from build123d import *

# Parameters (mm, degrees)
BOSS_EXTRU_1_DEPTH                              = 8
SKETCH1_R                                       = 3.375
CUT_EXTRUDE1_DEPTH                              = 9
ESQUISSE7_W                                     = 7
ESQUISSE7_H                                     = 3.5
ENL_V_MAT_EXTRU_2_DEPTH                         = 9
CHAMBRAGE_POUR_VIS_T_TE_CYLINDRIQUE_D           = 2.5
CHAMBRAGE_POUR_VIS_T_TE_CYLINDRIQUE_CBORE_D     = 4.5
CHAMBRAGE_POUR_VIS_T_TE_CYLINDRIQUE_CBORE_DEPTH = 5.3
CBORE_FOR_M5_HEX_HEAD_BOLT1_D                   = 4
CBORE_FOR_M5_HEX_HEAD_BOLT1_DEPTH               = 9.499
CBORE_FOR_M5_HEX_HEAD_BOLT1_CBORE_D             = 6.2
CBORE_FOR_M5_HEX_HEAD_BOLT1_CBORE_DEPTH         = 2
CBORE_FOR_M5_HEX_HEAD_BOLT1_TIP                 = 1.201721238


with BuildPart() as part:
    # Esquisse1 → Boss.-Extru.1 (new body)
    with BuildSketch(Plane(origin=(0, 0, 0), x_dir=(1, 0, 0), z_dir=(0, 1, 0))):
        with BuildLine():
            Line((6.025985397, 9.5), (-6.025985397, 9.5))
            ThreePointArc((-6.025985397, 9.5), (0, -11.25), (6.025985397, 9.5))
        make_face()
    extrude(amount=BOSS_EXTRU_1_DEPTH)

    # Sketch1 → Cut-Extrude1 (cut, through all)
    with BuildSketch(Plane(origin=(0, 8, 0), x_dir=(1, 0, 0), z_dir=(0, 1, 0))):
        Circle(SKETCH1_R)
    extrude(amount=-CUT_EXTRUDE1_DEPTH, mode=Mode.SUBTRACT)

    # Esquisse7 → Enlèv. mat.-Extru.2 (cut, through all)
    with BuildSketch(Plane(origin=(0, 8, 0), x_dir=(1, 0, 0), z_dir=(0, 1, 0))):
        with Locations((0, 5.75)):
            Rectangle(ESQUISSE7_W, ESQUISSE7_H)
    extrude(amount=-ENL_V_MAT_EXTRU_2_DEPTH, mode=Mode.SUBTRACT)

    # Chambrage pour vis à tête cylindrique à 6 pans creux (ou vis CHC) M21 (through all)
    with Locations(Plane(origin=(0, 8, 0), x_dir=(1, 0, 0), z_dir=(0, 1, 0))):
        with Locations((-8, 0), (0, -8), (8, 0)):
            CounterBoreHole(CHAMBRAGE_POUR_VIS_T_TE_CYLINDRIQUE_D / 2, CHAMBRAGE_POUR_VIS_T_TE_CYLINDRIQUE_CBORE_D / 2, CHAMBRAGE_POUR_VIS_T_TE_CYLINDRIQUE_CBORE_DEPTH)

    # CBORE for M5 Hex Head Bolt1
    with Locations(Plane(origin=(0, 0, -9.5), x_dir=(-1, 0, 0), z_dir=(0, 0, -1))):
        with Locations((0, 4)):
            CounterBoreHole(CBORE_FOR_M5_HEX_HEAD_BOLT1_D / 2, CBORE_FOR_M5_HEX_HEAD_BOLT1_CBORE_D / 2, CBORE_FOR_M5_HEX_HEAD_BOLT1_CBORE_DEPTH, depth=CBORE_FOR_M5_HEX_HEAD_BOLT1_DEPTH)
            with Locations((0, 0, -(CBORE_FOR_M5_HEX_HEAD_BOLT1_DEPTH + CBORE_FOR_M5_HEX_HEAD_BOLT1_TIP / 2))):  # 118° drill point
                Cone(0, CBORE_FOR_M5_HEX_HEAD_BOLT1_D / 2, CBORE_FOR_M5_HEX_HEAD_BOLT1_TIP, mode=Mode.SUBTRACT)


solid = part.part
Build history of the part. All positions in model axes, mm. A direction names the side the tool comes from. Coordinates: 2 decimals unless noted, no trailing zeros. Order: outer loops, then holes, each group sorted by start corner. A loop starts at its lowest first (then second) coordinate and runs counter-clockwise, first axis right, second up. Notation, with made-up numbers: (2, 17.5) - (38, 17.5) arc R25 ccw to (38, 46.5) - close; hole circle Ø7 at (13.5, 22). An arc over 180 degrees is marked (long way). Write each question's results on one line, items separated by ' | '. Start each with the question number.
Item 1: Flat gauge pins, fed straight in: pin 1 (3.5 mm diameter, centred on x = -7.5, z = 0.5, fed in from +Y); pin 2 (3 mm diameter, centred on x = 0, z = 8, fed in from +Y); pin 3 (2 mm diameter, centred on x = 4.5, y = 2, fed in from +Z); pin 4 (1 mm diameter, centred on y = 4, z = -5.5, fed in from -X). Where does each tip first touch, or does it go through?
Item 2: Band-saw the part on D-D on z = 2.75. Write the cut outline in (x, y), and give its area (3 significant figures).
Item 3: Wall check: probe 1 along Y at (x, z) = (-8.5, -1.75); probe 2 along Z at (x, y) = (-7, 7.5); probe 3 along Z at (x, y) = (10, 5.25). Give the ranges that are in metal, low to high. Write a range as [from, to].
Item 4: Band-saw the part on A-A on y = 7.5. Write the cut outline in (x, z) (3 decimals).
Item 5: Tool access for faces 5 (the face through (2, 0, 3)), 6 (the face through (-7, 2.7, 1)), 7 (the face through (0.672, 0.974, -8.514)), 8 (the face through (2, 8, 3)), 9 (the face through (-2, 7, -7.5)): list every direction of +Z, -Z, +X, -X, +Y, -Y with a clear straight run to the whole face (end or side of a thin tool).
Item 6: Mould opens along X. For faces 1 (the face through (-3, 6, -9.5)), 2 (the face through (-1, 6, -4)), 3 (the face through (1, 2.7, 9)), 4 (the face through (-0.406, 3.944, 11.243)) say: released by +X, released by -X, zero draft, split by the parting line, or undercut.
Item 7: Band-saw the part on C-C on y = 4.5. State how many separate pieces and enclosed holes the cut face has, and give its area (3 significant figures).
Item 8: Band-saw the part on B-B on x = 8. Write the cut outline in (y, z), and give its area (3 significant figures).
Numbers:
1) pin 1: y = 8 | pin 2: y = 2.7 | pin 3: z = 10.69 | pin 4: x = -10.08
2) outline: (-10.91, 0) - (-1.96, 0) - (-1.96, 8) - (-10.91, 8) - close; (1.96, 0) - (10.91, 0) - (10.91, 8) - (1.96, 8) - close | area: 143 mm^2
3) probe 1: [0, 2.7] | probe 2: [-8.81, -2.02], [2.02, 8.81] | probe 3: [-5.15, -1.03], [1.03, 5.15]
4) outline: (-6.026, -9.5) - (6.026, -9.5) arc R11.25 ccw (long way) to start; hole circle Ø4.5 at (-8, 0); hole (-3.5, -7.5) - (3.5, -7.5) - (3.5, -4) - (-3.5, -4) - close; hole circle Ø6.75 at (0, 0); hole circle Ø4.5 at (0, 8); hole circle Ø4.5 at (8, 0)
5) face 5: +Z, -Z, +X, -X, -Y | face 6: +Y | face 7: -Z | face 8: +Z, -Z, +X, -X, +Y | face 9: +Y, -Y
6) face 1: zero draft | face 2: undercut | face 3: undercut | face 4: split by the parting line
7) separate pieces: 1 | enclosed holes: 3 | area: 260 mm^2
8) outline: (0, -7.91) - (8, -7.91) - (8, -2.25) - (2.7, -2.25) - (2.7, -1.25) - (0, -1.25) - close; (0, 1.25) - (2.7, 1.25) - (2.7, 2.25) - (8, 2.25) - (8, 7.91) - (0, 7.91) - close | area: 96.0 mm^2
